```python
from build123d import *

# Parameters (mm, degrees)
BOSS_EXTRUDE1_DEPTH = 30
SKETCH3_W           = 20
SKETCH3_H           = 14
CUT_EXTRUDE1_DEPTH  = 60
BOSS_EXTRUDE2_DEPTH = 15
BOSS_EXTRUDE3_DEPTH = 6
CUT_EXTRUDE2_DEPTH  = 30


with BuildPart() as part:
    # Sketch2 → Boss-Extrude1 (new, symmetric)
    with BuildSketch(Plane.XY):
        Polygon((-9.659258263, 2.588190451), (0, 0), (31.058285412, 115.911099155), (21.399027149, 118.499289606), align=None)
    extrude(amount=BOSS_EXTRUDE1_DEPTH, both=True)

    # Sketch3 → Cut-Extrude1 (cut)
    with BuildSketch(Plane(origin=(0, 0, 0), x_dir=(0, 0, -1), z_dir=(0.9659258262890692, -0.25881904510251785, 0))):
        with Locations((-20, 97)):
            Rectangle(SKETCH3_W, SKETCH3_H)
        with Locations((-20, 67)):
            Rectangle(SKETCH3_W, SKETCH3_H)
    extrude(amount=-CUT_EXTRUDE1_DEPTH, mode=Mode.SUBTRACT)

    # Sketch5 → Boss-Extrude2 (add, symmetric)
    with BuildSketch(Plane(origin=(7.764571353, 28.977774789, 0), x_dir=(-0.9659258262890692, 0.25881904510251746, 0), z_dir=(-0.25881904510251746, -0.9659258262890692, 0))):
        Polygon((0, 24), (-54, 24), (-54, -65), (-60, -65), (-60, 30), (0, 30), align=None)
    extrude(amount=BOSS_EXTRUDE2_DEPTH, both=True)

    # Sketch6 → Boss-Extrude3 (add)
    with BuildSketch(Plane(origin=(57.955549577, -15.529142706, 0), x_dir=(0, 0, -1), z_dir=(0.9659258262890692, -0.25881904510251746, 0))):
        with BuildLine():
            Line((-65, 45), (-65, 15))
            ThreePointArc((-65, 15), (-80, 30), (-65, 45))
        make_face()
    extrude(amount=-BOSS_EXTRUDE3_DEPTH)

    # Sketch7 → Cut-Extrude2 (cut)
    with BuildSketch(Plane(origin=(57.955549577, -15.529142706, 0), x_dir=(0, 0, -1), z_dir=(0.9659258262890692, -0.25881904510251746, 0))):
        with BuildLine():
            Line((-65, 36), (-55, 36))
            ThreePointArc((-55, 36), (-49, 30), (-55, 24))
            Line((-55, 24), (-65, 24))
            ThreePointArc((-65, 24), (-71, 30), (-65, 36))
        make_face()
        with BuildLine():
            Line((-30, 36), (-20, 36))
            ThreePointArc((-20, 36), (-14, 30), (-20, 24))
            Line((-20, 24), (-30, 24))
            ThreePointArc((-30, 24), (-36, 30), (-30, 36))
        make_face()
        with BuildLine():
            Line((5, 36), (15, 36))
            ThreePointArc((15, 36), (21, 30), (15, 24))
            Line((15, 24), (5, 24))
            ThreePointArc((5, 24), (-1, 30), (5, 36))
        make_face()
    extrude(amount=-CUT_EXTRUDE2_DEPTH, mode=Mode.SUBTRACT)


solid = part.part
```
CAD build for the part. Positions are in the model's coordinates, mm. A direction names the side the tool comes from. Round coordinates to 2 decimals unless told otherwise and drop trailing zeros. Order: outer loops, then holes, each group sorted by start corner. A loop starts at its lowest first (then second) coordinate and runs counter-clockwise, first axis right, second up.
Item 1: Saw through at A-A on z = -7. Write the cut outline in (x, y).
Item 2: Saw through at C-C on z = 18.5. Write the cut outline in (x, y).
Item 3: Saw through at D-D on x = 25. Write the cut outline in (y, z).
Item 4: Saw through at B-B on z = 6. Write the cut outline in (x, y), then the cut area to 3 significant figures.
Item 5: Probe line 1 along Z through (x, y) = (57, 15); line 2 along Z through (x, y) = (-2.5, 14); line 3 along X through (y, z) = (53, -17.5). List the from-to ranges inside material, lowest first.
Item 6: Pin check, flat tips, straight feed: pin 1 (12.5 mm diameter, centred on x = 8.5, y = 19.5, fed in from +Z); pin 2 (10.5 mm diameter, centred on x = 14, y = 67, fed in from +Z); pin 3 (3 mm diameter, centred on x = 13.5, z = 14.5, fed in from +Y). Stop position of each tip, or through.
Item 7: Tool access for faces 5 (the face through (64.42, 20.01, 25.07)), 6 (the face through (10.77, 59.23, 20.14)), 7 (the face through (64.1, 29.41, -0.31)): list every direction of +Z, -Z, +X, -X, +Y, -Y with a clear straight run to the whole face (end or side of a thin tool).
Item 8: Mould opens along Y. For faces 1 (the face through (-4.897, 1.312, 0.42)), 2 (the face through (30, 37, -30)), 3 (the face through (62.8, 14.1, 1)), 4 (the face through (62.9, 14.3, -21)) say: pulls with the +Y half, pulls with the -Y half, needs draft (parallel to the pull), parting line crosses it, or undercut.
Reported:
1. outline: (-9.66, 2.59) - (0, 0) - (31.06, 115.91) - (21.4, 118.5) - close; (56.04, 0.51) - (61.84, -1.04) - (64.17, 7.65) - (58.37, 9.21) - close; (61.48, 20.8) - (67.27, 19.24) - (69.6, 27.94) - (63.81, 29.49) - close
2. outline: (-9.66, 2.59) - (0, 0) - (15.53, 57.96) - (5.87, 60.54) - close; (9.49, 74.07) - (19.15, 71.48) - (23.29, 86.93) - (13.63, 89.52) - close; (17.26, 103.04) - (26.92, 100.46) - (31.06, 115.91) - (21.4, 118.5) - close; (56.04, 0.51) - (61.84, -1.04) - (64.22, 7.84) - (58.42, 9.39) - close; (61.43, 20.61) - (67.22, 19.06) - (69.6, 27.94) - (63.81, 29.49) - close
3. outline: (8.83, -30) - (39.89, -30) - (39.89, -24) - (8.83, -24) - close; (93.3, -30) - (117.53, -30) - (117.53, 30) - (100.97, 30) - (100.97, 10) - (93.3, 10) - close
4. outline: (-9.66, 2.59) - (0, 0) - (31.06, 115.91) - (21.4, 118.5) - close; (56.04, 0.51) - (61.84, -1.04) - (69.6, 27.94) - (63.81, 29.49) - close
4. area: 1,380 mm2
5. line 1: z = -30 to -24
5. line 2: z = -30 to 30
5. line 3: x = 3.85 to 14.2
6. pin 1: stops at z = 30
6. pin 2: stops at z = 10
6. pin 3: stops at y = 89.52
7. face 5: none
7. face 6: +Z, +X
7. face 7: +Z, -Z, +X
8. face 1: pulls with the -Y half
8. face 2: needs draft
8. face 3: undercut
8. face 4: undercut
